Geometry: final body of the model. Coordinates: model frame, mm. Face numbers are marked on the shaded views. Round coordinates to 2 decimals unless told otherwise and drop trailing zeros. Order: outer loops, then holes, each group sorted by start corner. A loop starts at its lowest first (then second) coordinate and runs counter-clockwise, first axis right, second up. Notation, with made-up numbers: (55, -4) -> (61, -4) arc R18 cw to (61, 15) -> close; hole circle Ø10 at (-29, 69). An arc over 180 degrees is marked (long way). Put each result on its own line as item: value.
Autodesk Inventor part; units mm, degrees
ref_plane "YZ Plane" through (0, 0, 0) normal (1, 0, 0) x (0, 1, 0)
ref_plane "XZ Plane" through (0, 0, 0) normal (0, 1, 0) x (-1, 0, 0)
ref_plane "XY Plane" through (0, 0, 0) normal (0, 0, 1) x (1, 0, 0)
sketch "Sketch1" plane through (0, 0, 0) normal (0, 0, 1) x (1, 0, 0)
  line L0 (0, 0) -> (0, 43.5277) construction
  line L1 (0, 0) -> (22, 0)
  line L2 (22, 0) -> (22, 1.5)
  line L3 (22, 1.5) -> (20.4, 3.1)
  line L4 (20.4, 3.1) -> (22, 4.7)
  line L5 (22, 4.7) -> (22, 6.1)
  line L6 (22, 6.1) -> (27.5, 6.1)
  line L7 (27.5, 6.1) -> (27.5, 10.7)
  line L8 (27.5, 10.7) -> (25, 10.7)
  line L9 (25, 10.7) -> (25, 12.7)
  line L10 (25, 12.7) -> (28, 15.7)
  line L11 (25, 12.7) -> (29.2426, 12.7) construction
  line L12 (28, 15.7) -> (22.5, 15.7)
  line L13 (22.5, 15.7) -> (22.5, 8.6)
  line L14 (22.5, 8.6) -> (19.5, 8.6)
  line L15 (19.5, 8.6) -> (19.5, 0)
  dimension "d0" = 22
  dimension "d1" = 1.5
  dimension "d2" = 135
  dimension "d3" = 90
  dimension "d4" = 3.2
  dimension "d5" = 1.4
  dimension "d6" = 6.1
  dimension "d7" = 27.5
  dimension "d8" = 4.6
  dimension "d11" = 5
  dimension "d12" = 2.5
  dimension "d14" = 2.5
  dimension "d15" = 2.5
  dimension "d17" = 28
  dimension "d18" = 3
  dimension "d19" = 2
revolve "Revolution1" add sketch "Sketch1" angle 360 about axis through (0, 0, 0) along (0, 1, 0)
properties part number "101_Illumination_Adapter_Axiotech_COOLled"
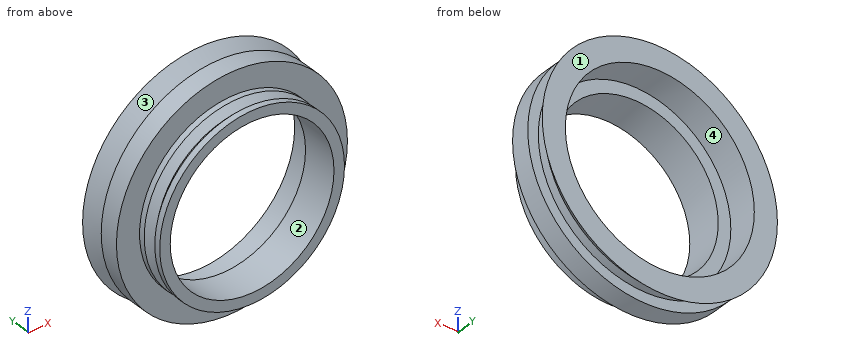
1. Cut plane B-B on x = 0. Return loops of the section in (y, z).
Ans:
outline: (0, -22) -> (1.5, -22) -> (3.1, -20.4) -> (4.7, -22) -> (6.1, -22) -> (6.1, -27.5) -> (10.7, -27.5) -> (10.7, -25) -> (12.7, -25) -> (15.7, -28) -> (15.7, -22.5) -> (8.6, -22.5) -> (8.6, -19.5) -> (0, -19.5) -> close; (0, 19.5) -> (8.6, 19.5) -> (8.6, 22.5) -> (15.7, 22.5) -> (15.7, 28) -> (12.7, 25) -> (10.7, 25) -> (10.7, 27.5) -> (6.1, 27.5) -> (6.1, 22) -> (4.7, 22) -> (3.1, 20.4) -> (1.5, 22) -> (0, 22) -> close
2. Cut plane A-A on z = 0. Return loops of the section in (x, y).
Ans:
outline: (-28, 15.7) -> (-25, 12.7) -> (-25, 10.7) -> (-27.5, 10.7) -> (-27.5, 6.1) -> (-22, 6.1) -> (-22, 4.7) -> (-20.4, 3.1) -> (-22, 1.5) -> (-22, 0) -> (-19.5, 0) -> (-19.5, 8.6) -> (-22.5, 8.6) -> (-22.5, 15.7) -> close; (19.5, 0) -> (22, 0) -> (22, 1.5) -> (20.4, 3.1) -> (22, 4.7) -> (22, 6.1) -> (27.5, 6.1) -> (27.5, 10.7) -> (25, 10.7) -> (25, 12.7) -> (28, 15.7) -> (22.5, 15.7) -> (22.5, 8.6) -> (19.5, 8.6) -> close
3. Contact query for flat-ended pins moving along their axis: P1, Ø10, axis at x = 14.5, z = 4, coming from the +Y side; P2, Ø1.5, axis at y = 2, z = -16.5, coming from the +X side; P3, Ø6, axis at x = 7, y = 9, coming from the +Z side. Output: stop coordinate, or through.
Ans:
P1: y = 8.6
P2: x = 15.16
P3: z = 27.21
4. Cut plane C-C on y = 9.5. Return loops of the section in (x, z).
Ans:
outline: circle Ø55 at (0, 0); hole circle Ø45 at (0, 0)
5. Draft query along X for the marked faces 1, 2, 3 and 4. Return one class per face: +X half, -X half, draft (parallel to the pull), parting line (faces both ways), or undercut.
Ans:
face 1: draft
face 2: undercut
face 3: parting line
face 4: undercut
6. Material intervals for probe 1 along X at (y, z) = (5.75, 0.5); probe 2 along Z at (x, y) = (0, 11.25), sorted ascending.
Ans:
probe 1: -21.99 to -19.49, 19.49 to 21.99
probe 2: -25 to -22.5, 22.5 to 25
